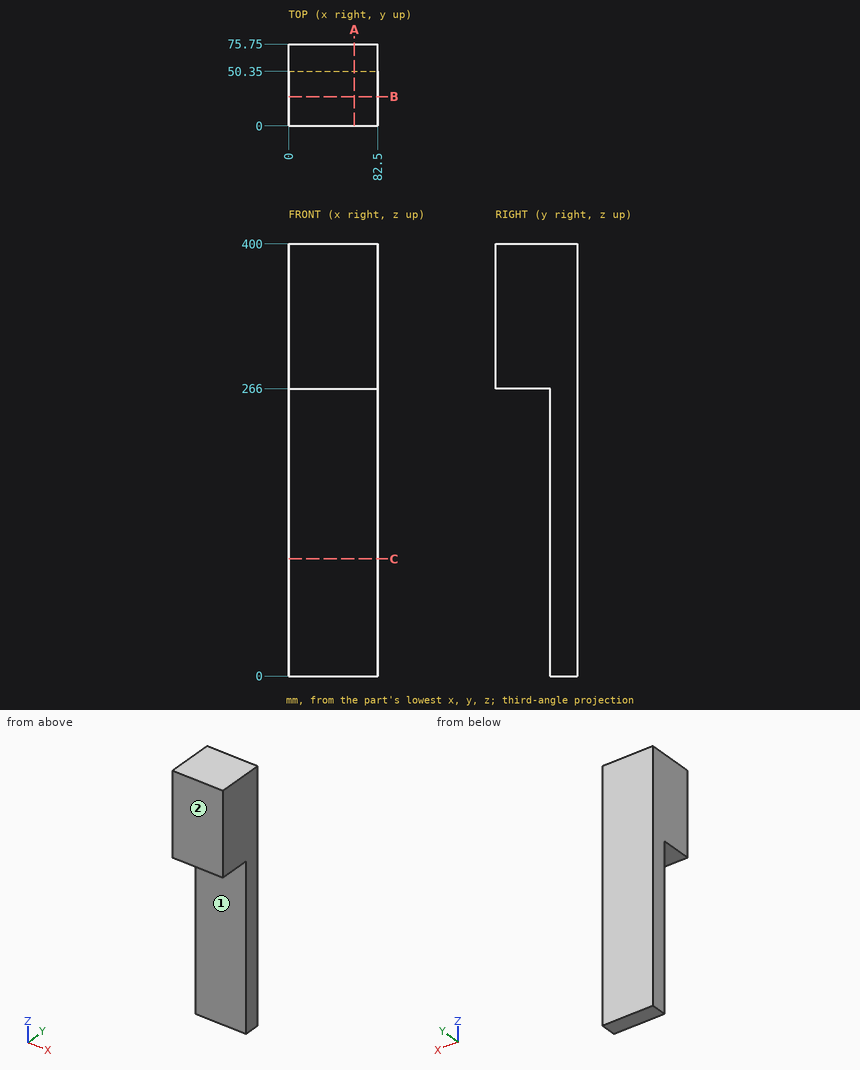
Job drawing, mm, ordinate dimensions from the low corner. One solid piece. A direction names the side the tool comes from. Coordinates: 2 decimals unless noted, no trailing zeros. Order: outer loops, then holes, each group sorted by start corner. A loop starts at its lowest first (then second) coordinate and runs counter-clockwise, first axis right, second up. Notation, with made-up numbers: (31, 0) - (80, 0) arc R33 cw to (80, 34) - close; hole circle Ø2 at (-37, -15.75). An arc over 180 degrees is marked (long way). Write each question's results on one line, items separated by ' | '. Start each with the question number.
Item 1: Tool access for the marked faces 1 and 2: list every direction of +Z, -Z, +X, -X, +Y, -Y with a clear straight run to the whole face (end or side of a thin tool).
Item 2: Band-saw the part on B-B on y = 27. Write the cut outline in (x, z), and give its area (3 significant figures).
Item 3: Flat gauge pin, fed straight in: pin 1 (25 mm diameter, centred on x = 26.5, y = 29.5, fed in from -Z). Where does the tip first touch, or does it go through?
Item 4: Wall check: probe 1 along Z at (x, y) = (54, 42); probe 2 along Y at (x, z) = (12.5, 217). Give the ranges that are in metal, low to high. Write a range as [from, to].
Item 5: Band-saw the part on C-C on z = 108.5. Write the cut outline in (x, y), and give its area (3 significant figures).
Item 6: Band-saw the part on A-A on x = 61. Write the cut outline in (y, z), and give its area (3 significant figures).
Numbers:
1) face 1: -Z, +X, -X, -Y | face 2: +Z, -Z, +X, -X, -Y
2) outline: (0, 266) - (82.5, 266) - (82.5, 400) - (0, 400) - close | area: 11,100 mm^2
3) pin 1: z = 266
4) probe 1: [266, 400] | probe 2: [50.35, 75.75]
5) outline: (0, 50.35) - (82.5, 50.35) - (82.5, 75.75) - (0, 75.75) - close | area: 2,100 mm^2
6) outline: (0, 266) - (50.35, 266) - (50.35, 0) - (75.75, 0) - (75.75, 400) - (0, 400) - close | area: 16,900 mm^2
